```python
from build123d import *

# Parameters (mm, degrees)
SKETCH1_W               = 63
SKETCH1_H               = 63
BOSS_EXTRUDE1_DEPTH     = 5
SKETCH3_W               = 63
SKETCH3_H               = 63
SKETCH3_W_2             = 60
SKETCH3_H_2             = 60
BOSS_EXTRUDE2_DEPTH     = 16
SKETCH7_W               = 250
SKETCH7_H               = 250
SKETCH7_W_2             = 60
SKETCH7_H_2             = 60
BOSS_EXTRUDE5_DEPTH     = 4
SKETCH9_W               = 250
SKETCH9_H               = 250
SKETCH9_W_2             = 210
SKETCH9_H_2             = 210
BOSS_EXTRUDE6_DEPTH     = 18
SKETCH10_W              = 222
SKETCH10_H              = 222
CUT_EXTRUDE1_DEPTH      = 4
SKETCH14_W              = 210
SKETCH14_H              = 210
SKETCH14_W_2            = 208
SKETCH14_H_2            = 208
BOSS_EXTRUDE9_DEPTH     = 14
SKETCH16_R              = 1.4
CUT_EXTRUDE2_DEPTH      = 10
MIRROR2_COPY_1_SKETCH_R = 1.4
MIRROR2_COPY_1_DEPTH    = 10
FILLET1_R               = 10
FILLET2_R               = 10
FILLET3_R               = 10
FILLET4_R               = 10
SKETCH17_W              = 63
SKETCH17_H              = 63
BOSS_EXTRUDE10_DEPTH    = 10
BOSS_EXTRUDE13_START    = -53
SKETCH18_W              = 69
SKETCH18_H              = 69
SKETCH18_W_2            = 63
SKETCH18_H_2            = 63
BOSS_EXTRUDE13_DEPTH    = 53
SKETCH20_W              = 69
SKETCH20_H              = 69
CUT_EXTRUDE3_DEPTH      = 18
SKETCH21_W              = 60
SKETCH21_H              = 60
CUT_EXTRUDE4_DEPTH      = 232.079018744
SKETCH24_W              = 76
SKETCH24_H              = 76
SKETCH24_W_2            = 69
SKETCH24_H_2            = 69
BOSS_EXTRUDE14_DEPTH    = 31
SKETCH25_R              = 1.4
CUT_EXTRUDE5_DEPTH      = 10
MIRROR4_COPY_1_SKETCH_R = 1.4
MIRROR4_COPY_1_DEPTH    = 10


with BuildPart() as part:
    # Sketch1 → Boss-Extrude1 (new body)
    with BuildSketch(Plane.XY):
        with Locations((-56.732567938, -12.574658475)):
            Rectangle(SKETCH1_W, SKETCH1_H)
    extrude(amount=BOSS_EXTRUDE1_DEPTH)

    # Sketch3 → Boss-Extrude2 (add)
    with BuildSketch(Plane.XY.offset(5)):
        with Locations((-56.732567938, -12.574658475)):
            Rectangle(SKETCH3_W, SKETCH3_H)
        with Locations((-56.732567938, -12.574658475)):
            Rectangle(SKETCH3_W_2, SKETCH3_H_2, mode=Mode.SUBTRACT)
    extrude(amount=BOSS_EXTRUDE2_DEPTH)

    # Sketch7 → Boss-Extrude5 (add)
    with BuildSketch(Plane.XY.offset(21)):
        with Locations((-56.732567938, -12.574658475)):
            Rectangle(SKETCH7_W, SKETCH7_H)
        with Locations((-56.732567938, -12.574658475)):
            Rectangle(SKETCH7_W_2, SKETCH7_H_2, mode=Mode.SUBTRACT)
    extrude(amount=BOSS_EXTRUDE5_DEPTH)

    # Sketch9 → Boss-Extrude6 (add)
    with BuildSketch(Plane.XY.offset(25)):
        with Locations((-56.732567938, -12.574658475)):
            Rectangle(SKETCH9_W, SKETCH9_H)
        with Locations((-56.732567938, -12.574658475)):
            Rectangle(SKETCH9_W_2, SKETCH9_H_2, mode=Mode.SUBTRACT)
    extrude(amount=BOSS_EXTRUDE6_DEPTH)

    # Sketch10 → Cut-Extrude1 (cut)
    with BuildSketch(Plane.XY.offset(43)):
        with Locations((-56.732567938, -12.574658475)):
            Rectangle(SKETCH10_W, SKETCH10_H)
    extrude(amount=-CUT_EXTRUDE1_DEPTH, mode=Mode.SUBTRACT)

    # Sketch14 → Boss-Extrude9 (add)
    with BuildSketch(Plane.XY.offset(25)):
        with Locations((-56.732567938, -12.574658475)):
            Rectangle(SKETCH14_W, SKETCH14_H)
        with Locations((-56.732567938, -12.574658475)):
            Rectangle(SKETCH14_W_2, SKETCH14_H_2, mode=Mode.SUBTRACT)
    extrude(amount=BOSS_EXTRUDE9_DEPTH)

    # Sketch16 → Cut-Extrude2 (cut)
    with BuildSketch(Plane.XY.offset(39)):
        with Locations((50.767432062, -120.074658475)):
            Circle(SKETCH16_R)
    cut_extrude2 = extrude(amount=-CUT_EXTRUDE2_DEPTH, mode=Mode.SUBTRACT)

    # Mirror1: Cut-Extrude2 across plane
    add(cut_extrude2.mirror(Plane(origin=(-56.732567938, 0, 0), x_dir=(0, 0, 1), z_dir=(1, 0, 0))), mode=Mode.SUBTRACT)

    # Mirror2: Cut-Extrude2 across plane
    add(cut_extrude2.mirror(Plane.ZX.offset(-12.574658475)), mode=Mode.SUBTRACT)

    # Mirror2 copy 1 sketch → Mirror2 copy 1 (cut)
    with BuildSketch(Plane(origin=(-113.465135876, -25.149316949, 39), x_dir=(-1, 0, 0), z_dir=(0, 0, 1))):
        with Locations((50.767432062, -120.074658475)):
            Circle(MIRROR2_COPY_1_SKETCH_R)
    extrude(amount=-MIRROR2_COPY_1_DEPTH, mode=Mode.SUBTRACT)

    # Fillet1
    fillet1_edges = [part.edges().sort_by_distance(p)[0] for p in [
        (-181.732567938, 112.425341525, 32),
    ]]
    fillet(fillet1_edges, radius=FILLET1_R)

    # Fillet2
    fillet2_edges = [part.edges().sort_by_distance(p)[0] for p in [
        (-181.732567938, -137.574658475, 32),
    ]]
    fillet(fillet2_edges, radius=FILLET2_R)

    # Fillet3
    fillet3_edges = [part.edges().sort_by_distance(p)[0] for p in [
        (68.267432062, 112.425341525, 32),
    ]]
    fillet(fillet3_edges, radius=FILLET3_R)

    # Fillet4
    fillet4_edges = [part.edges().sort_by_distance(p)[0] for p in [
        (68.267432062, -137.574658475, 32),
    ]]
    fillet(fillet4_edges, radius=FILLET4_R)

    # Sketch17 → Boss-Extrude10 (add)
    with BuildSketch(Plane(origin=(0, 0, 0), x_dir=(-1, 0, 0), z_dir=(0, 0, -1))):
        with Locations((56.732567938, -12.574658475)):
            Rectangle(SKETCH17_W, SKETCH17_H)
    extrude(amount=BOSS_EXTRUDE10_DEPTH)

    # Sketch18 → Boss-Extrude13 (add)
    with BuildSketch(Plane(origin=(0, 0, -10), x_dir=(-1, 0, 0), z_dir=(0, 0, -1)).offset(BOSS_EXTRUDE13_START)):
        with Locations((56.732567938, -12.574658475)):
            Rectangle(SKETCH18_W, SKETCH18_H)
        with Locations((56.732567938, -12.574658475)):
            Rectangle(SKETCH18_W_2, SKETCH18_H_2, mode=Mode.SUBTRACT)
    extrude(amount=BOSS_EXTRUDE13_DEPTH)

    # Sketch20 → Cut-Extrude3 (cut)
    with BuildSketch(Plane.XY.offset(43)):
        with Locations((-56.732567938, -12.574658475)):
            Rectangle(SKETCH20_W, SKETCH20_H)
    extrude(amount=-CUT_EXTRUDE3_DEPTH, mode=Mode.SUBTRACT)

    # Sketch21 → Cut-Extrude4 (cut, through all)
    with BuildSketch(Plane.XY.offset(5)):
        with Locations((-56.732567938, -12.574658475)):
            Rectangle(SKETCH21_W, SKETCH21_H)
    extrude(amount=-CUT_EXTRUDE4_DEPTH, mode=Mode.SUBTRACT)

    # Sketch24 → Boss-Extrude14 (add)
    with BuildSketch(Plane(origin=(0, 0, 21), x_dir=(-1, 0, 0), z_dir=(0, 0, -1))):
        with Locations((56.732567938, -12.574658475)):
            Rectangle(SKETCH24_W, SKETCH24_H)
        with Locations((56.732567938, -12.574658475)):
            Rectangle(SKETCH24_W_2, SKETCH24_H_2, mode=Mode.SUBTRACT)
    extrude(amount=BOSS_EXTRUDE14_DEPTH)

    # Sketch25 → Cut-Extrude5 (cut)
    with BuildSketch(Plane(origin=(0, 0, -10), x_dir=(-1, 0, 0), z_dir=(0, 0, -1))):
        with Locations((90.232567938, 20.925341525)):
            Circle(SKETCH25_R)
    cut_extrude5 = extrude(amount=-CUT_EXTRUDE5_DEPTH, mode=Mode.SUBTRACT)

    # Mirror3: Cut-Extrude5 across plane
    add(cut_extrude5.mirror(Plane.ZX.offset(-12.574658475)), mode=Mode.SUBTRACT)

    # Mirror4: Cut-Extrude5 across plane
    add(cut_extrude5.mirror(Plane.ZY.offset(56.732567938)), mode=Mode.SUBTRACT)

    # Mirror4 copy 1 sketch → Mirror4 copy 1 (cut)
    with BuildSketch(Plane(origin=(-113.465135876, -25.149316949, -10), x_dir=(1, 0, 0), z_dir=(0, 0, -1))):
        with Locations((90.232567938, 20.925341525)):
            Circle(MIRROR4_COPY_1_SKETCH_R)
    extrude(amount=-MIRROR4_COPY_1_DEPTH, mode=Mode.SUBTRACT)


solid = part.part
```
Work out the finished part from the listing and answer in its coordinate system (mm). A direction names the side the tool comes from. Round coordinates to 2 decimals unless told otherwise and drop trailing zeros. Write each loop counter-clockwise with the first axis right and the second up, starting at its lowest first coordinate (ties: lowest second). Pieces come first, ordered by that corner, then holes. Notation, with made-up numbers: (18, 0.5) - (29, 0.5) arc R13 cw to (29, 22.5) - close; hole circle Ø1 at (-18.75, 25). An arc over 180 degrees is marked (long way). Return JSON: item names as keys, results as strings. Group by question number.
Q1. Each of these flat-tipped pins is pushed along its axis until it touches: pin 1 Ø3.5 at (x, y) = (50.77, -120.07) entering from +Z; pin 2 Ø1.4 at (x, y) = (-23.5, -46) entering from -Z; pin 3 Ø1.7 at (x, y) = (50.77, 94.93) entering from -Z; pin 4 Ø4 at (x, z) = (-15.5, 17) entering from -Y. Where does it stop, or does it pass through?
Q2. The part is cut by section A-A on x = -30. Write down the section's boundary in (y, z), then the cut area to 3 significant figures.
Q3. The part is cut by section C-C on z = 9. Write down the section's boundary in (x, y).
Q4. The part is cut by section D-D on x = 26. Write down the section's boundary in (y, z).
Q5. The part is cut by section B-B on y = -24.5. Write down the section's boundary in (x, z).
Q6. For faces 1 (the flat face through (-57, 17.425, 7)), 2 (the flat face through (-56, -50.575, 6)), 3 (the flat face through (-18.733, -13, 6)), 4 (the flat face through (-58, 91.425, 32)), determine the directions among +Z, -Z, +X, -X, +Y, -Y from which every point of the face is accessible in a straight line to the end or side of a thin tool.
Q7. The mould has two halves that part along X. Classify faces 5 (the flat face through (-58, -137.575, 32)), 6 (the cylindrical face through (65.416, -134.568, 32.154)), 7 (the flat face through (-57, -42.575, 7)): released by +X, released by -X, zero draft, split by the parting line, or undercut.
Q8. Find the intervals of material crossed by L1, parallel to Y at x = -108.5, z = 28; L2, parallel to Y at x = -63.5, z = 41; L3, parallel to X at y = -7.5, z = 16, in increasing order.
Solved:
{
 "1": {"pin 1": "z = 39", "pin 2": "z = 0", "pin 3": "z = 21", "pin 4": "through"},
 "2": {"outline": "(-137.57, 21) - (-50.57, 21) - (-50.57, -10) - (-42.57, -10) - (-42.57, 25) - (-116.57, 25) - (-116.57, 39) - (-123.57, 39) - (-123.57, 43) - (-137.57, 43) - close; (17.43, -10) - (25.43, -10) - (25.43, 21) - (112.43, 21) - (112.43, 43) - (98.43, 43) - (98.43, 39) - (91.43, 39) - (91.43, 25) - (17.43, 25) - close", "area": "1,960 mm²"},
 "3": {"outline": "(-94.73, -50.57) - (-18.73, -50.57) - (-18.73, 25.43) - (-94.73, 25.43) - close; hole (-86.73, -42.57) - (-26.73, -42.57) - (-26.73, 17.43) - (-86.73, 17.43) - close"},
 "4": {"outline": "(-137.57, 21) - (112.43, 21) - (112.43, 43) - (98.43, 43) - (98.43, 39) - (91.43, 39) - (91.43, 25) - (-116.57, 25) - (-116.57, 39) - (-123.57, 39) - (-123.57, 43) - (-137.57, 43) - close"},
 "5": {"outline": "(-181.73, 21) - (-94.73, 21) - (-94.73, -10) - (-86.73, -10) - (-86.73, 25) - (-160.73, 25) - (-160.73, 39) - (-167.73, 39) - (-167.73, 43) - (-181.73, 43) - close; (-26.73, -10) - (-18.73, -10) - (-18.73, 21) - (68.27, 21) - (68.27, 43) - (54.27, 43) - (54.27, 39) - (47.27, 39) - (47.27, 25) - (-26.73, 25) - close"},
 "6": {"face 1": "+Z, -Z", "face 2": "-Z, +X, -X, -Y", "face 3": "-Z, +X, +Y, -Y", "face 4": "+Z"},
 "7": {"face 5": "zero draft", "face 6": "released by +X", "face 7": "undercut"},
 "8": {"L1": "-137.57 to -116.57, 91.43 to 112.43", "L2": "-137.57 to -123.57, 98.43 to 112.43", "L3": "-94.73 to -86.73, -26.73 to -18.73"}
}
